Source: three-view drawing plus pictorial views. Frame: mm from the lowest corner of the part. Round coordinates to 2 decimals unless told otherwise and drop trailing zeros. Loops run counter-clockwise (first coordinate to the right, second up) from the corner with the lowest first, then second, coordinate; pieces in that order, holes last. Notation, with made-up numbers: M 56.25,-35 L 106.25,-35 A26 cw 106.25,-2 Z; hole C 51.5,77 d11. An arc over 180 degrees is marked long. Return JSON: item names as keys, results as strings. Group by question number.
1) Material intervals for line 1 (X direction, y = 135, z = 4); line 2 (Y direction, x = 80.5, z = 4.5); line 3 (X direction, y = 32, z = 2), sorted ascending. Write a range as from..to.
2) Contact query for flat-ended pins moving along their axis: P1, Ø4.5, axis at x = 75, y = 125, coming from the +Z side; P2, Ø2, axis at x = 64.5, z = 2, coming from the -Y side; P3, Ø1.5, axis at y = 131, z = 3.5, coming from the -X side; P4, Ø2, axis at x = 84.5, z = 5, coming from the +Y side. Output: stop coordinate, or through.
3) Section B-B (y = 115). Output: boundary loops of the cut face in (x, z).
4) Section C-C (y = 145). Output: boundary loops of the cut face in (x, z).
5) Section A-A (z = 1). Output: boundary loops of the cut face in (x, y), plus the area to 3 significant figures.
6) Section D-D (x = 17). Output: boundary loops of the cut face in (y, z), plus the area to 3 significant figures.
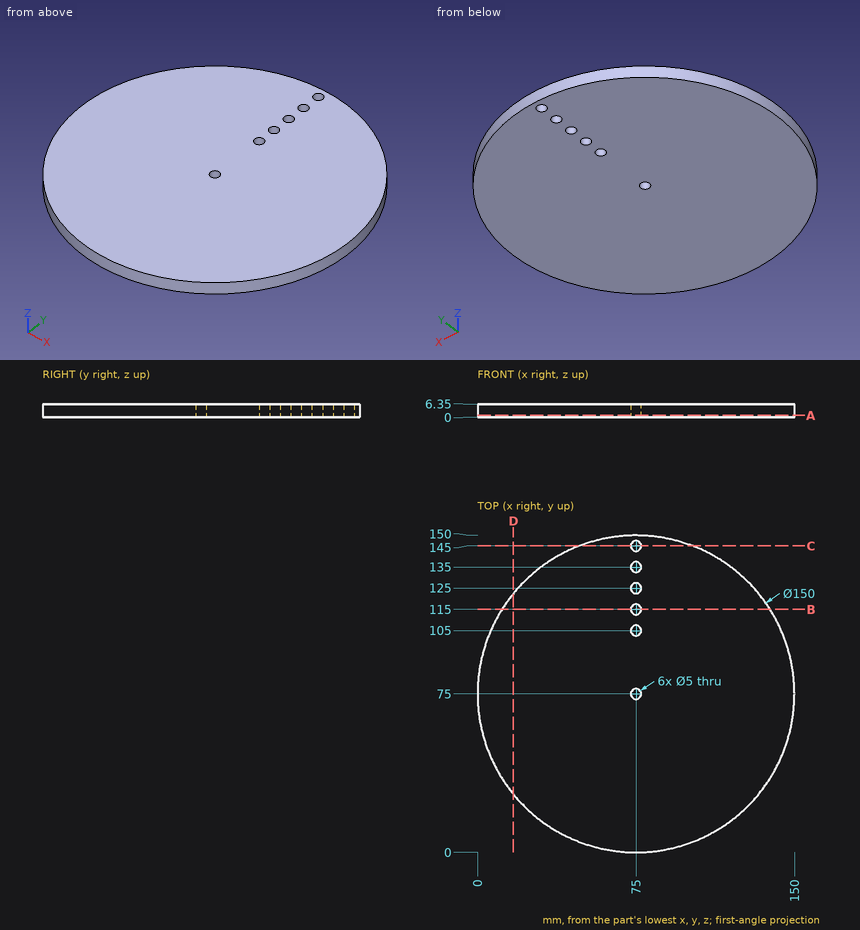
Returned:
{
 "1": {"line 1": "x = 30..72.5, 77.5..120", "line 2": "y = 0.2..149.8", "line 3": "x = 13.55..136.45"},
 "2": {"P1": "passes through", "P2": "stops at y = 0.6", "P3": "stops at x = 24.28", "P4": "stops at y = 149.52"},
 "3": {"outline": "M 11.56,0 L 72.5,0 L 72.5,6.35 L 11.56,6.35 Z; M 77.5,0 L 138.44,0 L 138.44,6.35 L 77.5,6.35 Z"},
 "4": {"outline": "M 48.07,0 L 72.5,0 L 72.5,6.35 L 48.07,6.35 Z; M 77.5,0 L 101.93,0 L 101.93,6.35 L 77.5,6.35 Z"},
 "5": {"outline": "C 75,75 d150; hole C 75,75 d5; hole C 75,105 d5; hole C 75,115 d5; hole C 75,125 d5; hole C 75,135 d5; hole C 75,145 d5", "area": "17,600 mm^2"},
 "6": {"outline": "M 27.45,0 L 122.55,0 L 122.55,6.35 L 27.45,6.35 Z", "area": "604 mm^2"}
}
